The model under review builds one solid part; all positions refer to its coordinate system, in mm. A direction names the side the tool comes from. Give positions to 0.01 mm unless a question says otherwise; leave off trailing zeros. Loops run counter-clockwise (first coordinate to the right, second up) from the corner with the lowest first, then second, coordinate; pieces in that order, holes last. Notation, with made-up numbers: (65.5, 70.5) - (72.5, 70.5) arc R25 ccw to (72.5, 84.5) - close; hole circle Ø2 at (-7, 65.25). An arc over 180 degrees is marked (long way). Answer as a JSON object with one key per item and string values.
from build123d import *

# Parameters (mm, degrees)
SKETCH1_R           = 4.5
BOSS_EXTRUDE1_DEPTH = 15
CUT_EXTRUDE1_DEPTH  = 15
CIRPATTERN1_COUNT   = 4


with BuildPart() as part:
    # Sketch1 → Boss-Extrude1 (new body)
    with BuildSketch(Plane(origin=(0, 0, 0), x_dir=(1, 0, 0), z_dir=(0, 1, 0))):
        Circle(SKETCH1_R)
    extrude(amount=BOSS_EXTRUDE1_DEPTH)

    # Sketch2 → Cut-Extrude1 (cut)
    with BuildSketch(Plane(origin=(0, 15, 0), x_dir=(1, 0, 0), z_dir=(0, 1, 0))):
        with BuildLine():
            Line((-1.436091353, 4.264697132), (-1.002466053, 3.353365744))
            ThreePointArc((-1.002466053, 3.353365744), (-0.040083536, 3.499770465), (0.925399693, 3.375445957))
            Line((0.925399693, 3.375445957), (1.52547781, 4.233546675))
            ThreePointArc((1.52547781, 4.233546675), (0.047329403, 4.499751096), (-1.436091353, 4.264697132))
        make_face()
    cut_extrude1 = extrude(amount=-CUT_EXTRUDE1_DEPTH, mode=Mode.SUBTRACT)

    # CirPattern1: Cut-Extrude1 ×4 about axis
    cirpattern1_axis = Axis((0, 0, 0), (0, 1, 0))
    for i in range(1, CIRPATTERN1_COUNT):
        add(cut_extrude1.rotate(cirpattern1_axis, i * 360 / CIRPATTERN1_COUNT), mode=Mode.SUBTRACT)


solid = part.part
Q1. For faces 4 (the face through (1.222, 7.605, 3.815)), 5 (the face through (-3.8, 7.6, -1.22)), 6 (the face through (1.22, 7.6, -3.8)), list the 3-axis set-ups (+Z, -Z, +X, -X, +Y, -Y) from which the entire face can be reached by the end or side of a thin tool; tool diameter is ignored.
Results:
{"face 4": "+Z, +Y, -Y", "face 5": "-X, +Y, -Y", "face 6": "-Z, +Y, -Y"}
Q2. Consider section B-B, the plane x = 0. State the section outline as (y, z) points.
Results:
{"outline": "(0, -3.5) - (15, -3.5) - (15, 3.5) - (0, 3.5) - close"}
Q3. Consider section C-C, the plane z = 1.75. State the section outline as (x, y) points.
Results:
{"outline": "(-4.15, 0) - (4.15, 0) - (4.15, 15) - (-4.15, 15) - close"}
Q4. Clearance check with flat-ended pins moving along their axes: pin 1 Ø5 at (x, y) = (1.5, 6) entering from -Z; pin 2 Ø1.5 at (y, z) = (2.5, 1) entering from +X; pin 3 Ø1.5 at (x, y) = (2.5, 6) entering from +Z. State where each tip first meets the part, or that it passes through.
Results:
{"pin 1": "stops at z = -4.23", "pin 2": "stops at x = 4.23", "pin 3": "stops at z = 4.15"}
Q5. Consider section A-A, the plane y = 6. State the section outline as (x, z) points.
Results:
{"outline": "(-4.26, 1.44) - (-3.35, 1) arc R3.5 ccw to (-3.38, -0.93) - (-4.23, -1.53) arc R4.5 ccw to (-1.44, -4.26) - (-1, -3.35) arc R3.5 ccw to (0.93, -3.38) - (1.53, -4.23) arc R4.5 ccw to (4.26, -1.44) - (3.35, -1) arc R3.5 ccw to (3.38, 0.93) - (4.23, 1.53) arc R4.5 ccw to (1.44, 4.26) - (1, 3.35) arc R3.5 ccw to (-0.93, 3.38) - (-1.53, 4.23) arc R4.5 ccw to start"}
Q6. To check wall thickness, follow probe 1 along X at (y, z) = (7, 0); probe 2 along X at (y, z) = (1, 3.75); probe 3 along Z at (x, y) = (-3, 2.75). State the ranges of each line that lie inside material, in increasing order. Write a range as [from, to].
Results:
{"probe 1": "x = [-3.5, 3.5]", "probe 2": "x = [-2.49, -1.19], [1.19, 2.49]", "probe 3": "z = [-3.35, 3.35]"}
Q7. The part is to be moulded in two halves that separate along Z. For faces 1 (the face through (3.5, 7.6, -0.1)), 2 (the face through (-3.235, 7.395, 3.128)), 3 (the face through (0, 0, 0)), say which applies: +Z half, -Z half, draft (parallel to the pull), parting line (faces both ways), or undercut.
Results:
{"face 1": "undercut", "face 2": "+Z half", "face 3": "draft"}
